Source: three-view drawing plus pictorial views. Frame: mm from the lowest corner of the part. A direction names the side the tool comes from. Coordinates: 2 decimals unless noted, no trailing zeros. Order: outer loops, then holes, each group sorted by start corner. A loop starts at its lowest first (then second) coordinate and runs counter-clockwise, first axis right, second up. Notation, with made-up numbers: (-10, 25.5) - (25, 25.5) arc R26 ccw to (25, 42.5) - close; hole circle Ø4 at (64, -35.5). An arc over 180 degrees is marked (long way). One line per question, with ' | ' between items.
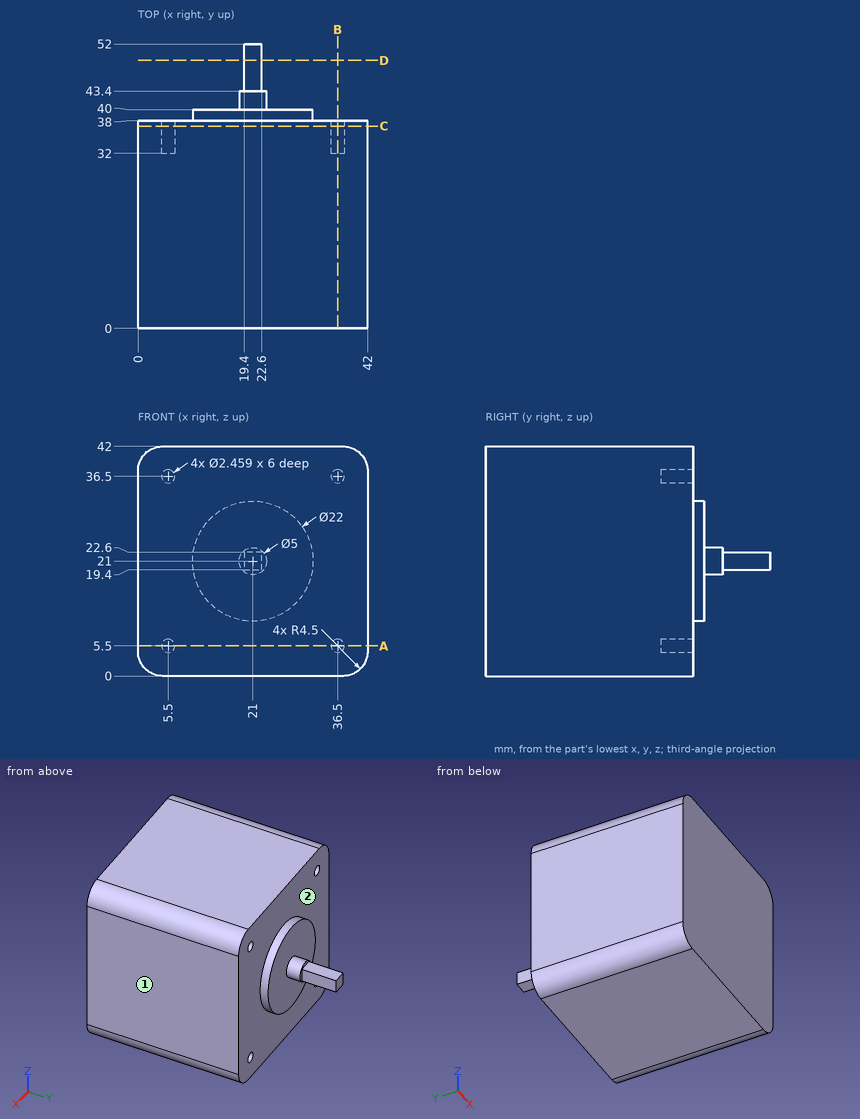
(1) Cut plane A-A (z = 5.5). Return the cut outline in (x, y).
Taken from the geometry:
outline: (0, 0) - (42, 0) - (42, 38) - (37.73, 38) - (37.73, 32) - (35.27, 32) - (35.27, 38) - (6.73, 38) - (6.73, 32) - (4.27, 32) - (4.27, 38) - (0, 38) - close
(2) Cut plane C-C (y = 37). Return the cut outline in (x, z), and give its area (3 significant figures).
Taken from the geometry:
outline: (0, 4.5) arc R4.5 ccw to (4.5, 0) - (37.5, 0) arc R4.5 ccw to (42, 4.5) - (42, 37.5) arc R4.5 ccw to (37.5, 42) - (4.5, 42) arc R4.5 ccw to (0, 37.5) - close; hole circle Ø2.46 at (5.5, 5.5); hole circle Ø2.46 at (5.5, 36.5); hole circle Ø2.46 at (36.5, 5.5); hole circle Ø2.46 at (36.5, 36.5) | area: 1,730 mm²
(3) Set-up query: the marked faces 1 and 2. Return all of +Z, -Z, +X, -X, +Y, -Y with unobstructed straight access to the full face (end or side cutting, diameter ignored); none if empty.
Taken from the geometry:
face 1: +Z, -Z, +X, +Y, -Y | face 2: +Y
(4) Pin query (flat end, axial travel): P1, Ø3, axis at x = 5.5, z = 36.5, coming from the +Y side; P2, Ø0.7, axis at x = 5.5, z = 36.5, coming from the +Y side; P3, Ø2.5, axis at x = 21.5, y = 47.5, coming from the -Z side; P4, Ø6, axis at y = 21, z = 28.5, coming from the -X side. Return the tip coordinate at first contact, or that it passes through.
Taken from the geometry:
P1: stops at y = 38 | P2: stops at y = 32 | P3: stops at z = 19.4 | P4: stops at x = 0
(5) Material intervals for L1, parallel to X at y = 36.15, z = 5.5; L2, parallel to X at y = 36, z = 5, sorted ascending. Write a range as from..to.
Taken from the geometry:
L1: x = 0..4.27, 6.73..35.27, 37.73..42 | L2: x = 0..4.38, 6.62..35.38, 37.62..42
(6) Cut plane D-D (y = 49). Return the cut outline in (x, z), and give its area (3 significant figures).
Taken from the geometry:
outline: (19.4, 19.4) - (22.6, 19.4) - (22.6, 22.6) - (19.4, 22.6) - close | area: 10.2 mm²
(7) Cut plane B-B (x = 36.5). Return the cut outline in (y, z).
Taken from the geometry:
outline: (0, 0) - (38, 0) - (38, 4.27) - (32, 4.27) - (32, 6.73) - (38, 6.73) - (38, 35.27) - (32, 35.27) - (32, 37.73) - (38, 37.73) - (38, 42) - (0, 42) - close
